Source: CAD feature listing. Evaluate the final solid. Frame: model axes, mm. Round coordinates to 2 decimals unless told otherwise and drop trailing zeros. Order: outer loops, then holes, each group sorted by start corner. A loop starts at its lowest first (then second) coordinate and runs counter-clockwise, first axis right, second up. Notation, with made-up numbers: (-20.75, -21) -> (12.25, -21) arc R21 ccw to (12.25, 12) -> close; hole circle Ø5 at (-23, 45). An arc over 180 degrees is marked (long way). Answer as CSV lines item,"result".
from build123d import *

# Parameters (mm, degrees)
SKETCH1_R           = 3.175
BOSS_EXTRUDE1_DEPTH = 3.175


with BuildPart() as part:
    # Sketch1 → Boss-Extrude1 (new body)
    with BuildSketch(Plane.XY):
        with BuildLine():
            Line((18.052936785, 76.341523137), (-42.240313215, 63.554909137))
            ThreePointArc((-42.240313215, 63.554909137), (-49.473481519, 59.125864726), (-52.305574358, 51.131216))
            Line((-52.305574358, 51.131216), (-52.305574358, 0))
            Line((-52.305574358, 0), (33.387675642, 0))
            Line((33.387675642, 0), (33.387675642, 63.91783))
            ThreePointArc((33.387675642, 63.91783), (28.682324369, 73.785737161), (18.052936785, 76.341523137))
        make_face()
        with Locations((20.687675642, 20.35683)):
            Circle(SKETCH1_R, mode=Mode.SUBTRACT)
        with Locations((20.687675642, 63.91783)):
            Circle(SKETCH1_R, mode=Mode.SUBTRACT)
        with Locations((-8.776324358, 20.35683)):
            Circle(SKETCH1_R, mode=Mode.SUBTRACT)
        with Locations((-39.605574358, 51.131216)):
            Circle(SKETCH1_R, mode=Mode.SUBTRACT)
    extrude(amount=BOSS_EXTRUDE1_DEPTH)


solid = part.part
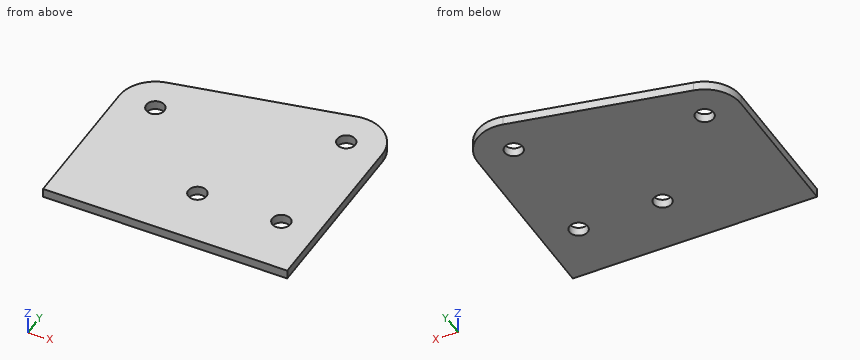
1. Section query A-A on z = 1.2. Return loops of the section in (x, y) (3 decimals).
Results below:
outline,"(-52.306, 0) -> (33.388, 0) -> (33.388, 63.918) arc R12.7 ccw to (18.053, 76.342) -> (-42.24, 63.555) arc R12.7 ccw to (-52.306, 51.131) -> close; hole circle Ø6.35 at (-39.606, 51.131); hole circle Ø6.35 at (-8.776, 20.357); hole circle Ø6.35 at (20.688, 20.357); hole circle Ø6.35 at (20.688, 63.918)"
2. Section query C-C on x = -18.5. Return loops of the section in (y, z) (3 decimals), and give its area (3 significant figures).
Results below:
outline,"(0, 0) -> (68.59, 0) -> (68.59, 3.175) -> (0, 3.175) -> close"
area,"218 mm2"
3. Line query: L1, parallel to Y at x = 22.5, z = 0.4; L2, parallel to X at y = 18.5, z = 0.7; L3, parallel to X at y = 21.5, z = 3. Output: solid intervals per line, ascending. Write a range as [from, to].
Results below:
L1,"[0, 17.75], [22.96, 61.31], [66.52, 76.49]"
L2,"[-52.31, -11.35], [-6.2, 18.11], [23.26, 33.39]"
L3,"[-52.31, -11.74], [-5.81, 17.73], [23.65, 33.39]"
4. Section query B-B on x = -7.5. Return loops of the section in (y, z) (3 decimals).
Results below:
outline,"(0, 0) -> (17.45, 0) -> (17.45, 3.175) -> (0, 3.175) -> close; (23.264, 0) -> (70.922, 0) -> (70.922, 3.175) -> (23.264, 3.175) -> close"
